For this review, take the finished solid that the model builds, in its own axes (mm). Face numbers are marked on the shaded views. A direction names the side the tool comes from. Coordinates: 2 decimals unless noted, no trailing zeros. Write each loop counter-clockwise with the first axis right and the second up, starting at its lowest first coordinate (ties: lowest second). Pieces come first, ordered by that corner, then holes.
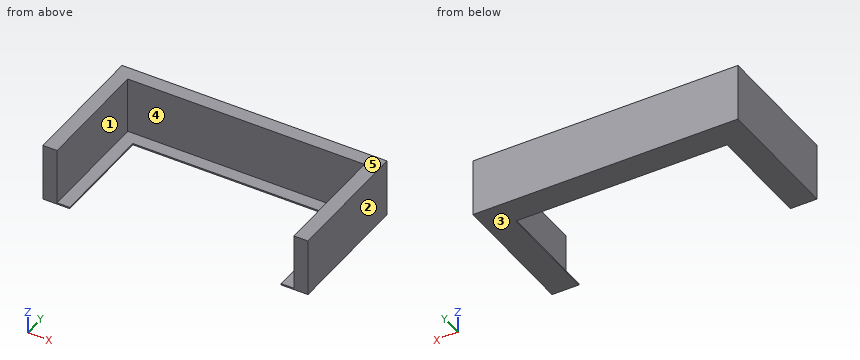
Autodesk Inventor part; units mm, degrees
ref_plane "YZ Plane" through (0, 0, 0) normal (1, 0, 0) x (0, 1, 0)
ref_plane "XZ Plane" through (0, 0, 0) normal (0, 1, 0) x (-1, 0, 0)
ref_plane "XY Plane" through (0, 0, 0) normal (0, 0, 1) x (1, 0, 0)
sketch "Sketch1" plane through (0, 0, 0) normal (0, 0, 1) x (1, 0, 0)
  line L0 (-273.8289, 101.7521) -> (-188.1039, 101.7521) construction
  line L1 (-188.1039, 101.7521) -> (-188.1039, 47.7771) construction
  line L2 (-188.1039, 47.7771) -> (-273.8289, 47.7771) construction
  line L3 (-273.8289, 47.7771) -> (-273.8289, 101.7521) construction
  line L4 (-343.37, 152.3416) -> (456.63, 152.3416) construction
  line L5 (456.63, 152.3416) -> (456.63, -1269.8807) construction
  line L6 (456.63, -1269.8807) -> (-343.37, -1269.8807) construction
  line L7 (-343.37, -1269.8807) -> (-343.37, 152.3416) construction
  line L8 (0, 0) -> (0, 158) construction
  line L9 (0, 158) -> (158, 158) construction
  line L10 (158, 158) -> (158, 0) construction
  line L11 (158, 0) -> (0, 0) construction
  line L12 (26, 26) -> (26, 132) construction
  line L13 (26, 132) -> (132, 132) construction
  line L14 (132, 132) -> (132, 26) construction
  line L15 (132, 26) -> (26, 26) construction
  line L16 (0, 158) -> (158, 0) construction
  line L17 (26, 26) -> (132, 132) construction
  line L18 (-5, 163) -> (163, 163)
  line L19 (163, 163) -> (163, 79)
  line L20 (163, 79) -> (-5, 79)
  line L21 (-5, 79) -> (-5, 163)
  line L22 (-15, 173) -> (173, 173)
  line L23 (173, 173) -> (173, 79)
  line L24 (173, 79) -> (-15, 79)
  line L25 (-15, 79) -> (-15, 173)
  line L26 (4, 154) -> (154, 154)
  line L27 (154, 154) -> (154, 79)
  line L28 (154, 79) -> (4, 79)
  line L29 (4, 79) -> (4, 154)
  point P0 (79, 79)
  point P1 (4, 79)
  point P2 (163, 79)
  point P3 (163, 79)
  dimension "d1" = 85.725
  dimension "d2" = 53.975
  dimension "d43" = 800.0001
  dimension "d52" = 158
  dimension "d53" = 158
  dimension "d59" = 106
  dimension "d60" = 106
  dimension "d62" = 5
  dimension "d63" = 5
  dimension "d64" = 5
  dimension "d65" = 10
  dimension "d66" = 10
  dimension "d67" = 10
  dimension "d68" = 4
  dimension "d69" = 4
  dimension "d70" = 4
extrude "Extrusion1" add sketch "Sketch1" against normal blind 1 contours L21 L24 L25 L22 L23 L19 L18 | L18 L19 L20 L27 L26 L29 L21
extrude "Extrusion2" add sketch "Sketch1" along normal blind 40 contours L21 L24 L25 L22 L23 L19 L18
properties part number "DoorButtonMount"
1) Consider section C-C (x = 102). Give the boundary of the cut face in (y, z), then the cut area to 3 significant figures.
2) Tool access review of the marked faces 4 and 5: name each direction out of +Z, -Z, +X, -X, +Y, -Y from which nothing blocks a thin tool from reaching the whole face with its end or side.
3) The part is to be moulded in two halves that separate along X. For the marked faces 1, 2 and 3, say which applies: pulls with the +X half, pulls with the -X half, needs draft (parallel to the pull), parting line crosses it, or undercut.
4) Consider section B-B (z = 16). Give the boundary of the cut face in (x, y).
5) Clearance check with flat-ended pins moving along their axes: P1, Ø2, axis at x = 95.5, z = 28, coming from the -Y side; P2, Ø1.1, axis at x = 66.5, z = -0.5, coming from the -Y side. State where each tip first meets the part, or that it passes through.
6) Consider section A-A (y = 147). Give the boundary of the cut face in (x, z).
7) For L1, parallel to X at y = 95.5, z = 11.5; L2, parallel to Y at x = 62, z = 28; L3, parallel to Z at x = -0.5, y = 129.5, list the stretches that pass through material, from the lowest coordinate up.
Results:
1. outline: (154, -1) - (173, -1) - (173, 40) - (163, 40) - (163, 0) - (154, 0) - close
1. area: 419 mm2
2. face 4: +Z, -Y
2. face 5: +Z, +X, -X, +Y, -Y
3. face 1: undercut
3. face 2: pulls with the +X half
3. face 3: needs draft
4. outline: (-15, 79) - (-5, 79) - (-5, 163) - (163, 163) - (163, 79) - (173, 79) - (173, 173) - (-15, 173) - close
5. P1: stops at y = 163
5. P2: stops at y = 154
6. outline: (-15, -1) - (4, -1) - (4, 0) - (-5, 0) - (-5, 40) - (-15, 40) - close; (154, -1) - (173, -1) - (173, 40) - (163, 40) - (163, 0) - (154, 0) - close
7. L1: x = -15 to -5, 163 to 173
7. L2: y = 163 to 173
7. L3: z = -1 to 0
